```python
from build123d import *

# Parameters (mm, degrees)
BOX004_W          = 49.8
BOX004_H          = 30
BOX004_DEPTH      = 20
CYLINDER001_R     = 2
CYLINDER001_DEPTH = 54
CYLINDER_R        = 2
CYLINDER_DEPTH    = 54
BOX003_W          = 54
BOX003_H          = 30
BOX003_DEPTH      = 20
FILLET003_R       = 2
FILLET004_R       = 2
BOX002_W          = 30
BOX002_H          = 20
BOX002_DEPTH      = 2
FILLET002_R       = 3
BOX001_W          = 30
BOX001_H          = 40
BOX001_DEPTH      = 2
FILLET001_R       = 3
BOX_W             = 50
BOX_H             = 100
BOX_DEPTH         = 2
FILLET_R          = 3


with BuildPart() as cub004:
    # Box004 → Box004 (new body)
    with BuildSketch(Plane(origin=(2.1, 0, 0), x_dir=(1, 0, 0), z_dir=(0, 0, 1))):
        with Locations((24.9, 15)):
            Rectangle(BOX004_W, BOX004_H)
    extrude(amount=BOX004_DEPTH)


with BuildPart() as cilindre001:
    # Cylinder001 → Cylinder001 (new body)
    with BuildSketch(Plane(origin=(0, 23, 11), x_dir=(0, 0, -1), z_dir=(1, 0, 0))):
        Circle(CYLINDER001_R)
    extrude(amount=CYLINDER001_DEPTH)


with BuildPart() as cilindre:
    # Cylinder → Cylinder (new body)
    with BuildSketch(Plane(origin=(0, 7, 11), x_dir=(0, 0, -1), z_dir=(1, 0, 0))):
        Circle(CYLINDER_R)
    extrude(amount=CYLINDER_DEPTH)


with BuildPart() as fillet004:
    # Box003 → Box003 (new body)
    with BuildSketch(Plane.XY):
        with Locations((27, 15)):
            Rectangle(BOX003_W, BOX003_H)
    extrude(amount=BOX003_DEPTH)

    # Cut002: cut Cilindre
    add(cilindre.part, mode=Mode.SUBTRACT)

    # Cut003: cut Cilindre001
    add(cilindre001.part, mode=Mode.SUBTRACT)

    # Cut004: cut Cub004
    add(cub004.part, mode=Mode.SUBTRACT)

    # Fillet003
    fillet003_edges = [fillet004.edges().sort_by_distance(p)[0] for p in [
        (54, 15, 0),
    ]]
    fillet(fillet003_edges, radius=FILLET003_R)

    # Fillet004
    fillet004_edges = [fillet004.edges().sort_by_distance(p)[0] for p in [
        (0, 15, 0),
    ]]
    fillet(fillet004_edges, radius=FILLET004_R)


with BuildPart() as fillet004_1:
    # Fillet004 placement: moved
    add(fillet004.part.moved(Location((-2, 0, 0))))


with BuildPart() as fillet002:
    # Box002 → Box002 (new body)
    with BuildSketch(Plane(origin=(10, 70, 0), x_dir=(1, 0, 0), z_dir=(0, 0, 1))):
        with Locations((15, 10)):
            Rectangle(BOX002_W, BOX002_H)
    extrude(amount=BOX002_DEPTH)

    # Fillet002
    fillet002_edges = [fillet002.edges().sort_by_distance(p)[0] for p in [
        (10, 70, 1),
        (10, 90, 1),
        (40, 70, 1),
        (40, 90, 1),
    ]]
    fillet(fillet002_edges, radius=FILLET002_R)


with BuildPart() as fillet001:
    # Box001 → Box001 (new body)
    with BuildSketch(Plane(origin=(10, 10, 0), x_dir=(1, 0, 0), z_dir=(0, 0, 1))):
        with Locations((15, 20)):
            Rectangle(BOX001_W, BOX001_H)
    extrude(amount=BOX001_DEPTH)

    # Fillet001
    fillet001_edges = [fillet001.edges().sort_by_distance(p)[0] for p in [
        (10, 10, 1),
        (10, 50, 1),
        (40, 10, 1),
        (40, 50, 1),
    ]]
    fillet(fillet001_edges, radius=FILLET001_R)


with BuildPart() as fusion001:
    # Box → Box (new body)
    with BuildSketch(Plane.XY):
        with Locations((25, 50)):
            Rectangle(BOX_W, BOX_H)
    extrude(amount=BOX_DEPTH)

    # Fillet
    fillet_edges = [fusion001.edges().sort_by_distance(p)[0] for p in [
        (0, 100, 1),
        (50, 100, 1),
    ]]
    fillet(fillet_edges, radius=FILLET_R)

    # Cut: cut Fillet001
    add(fillet001.part, mode=Mode.SUBTRACT)

    # Cut001: cut Fillet002
    add(fillet002.part, mode=Mode.SUBTRACT)

    # Fusion: union Fillet004
    add(fillet004_1.part)


solid = fusion001.part
```
Build history of the part. All positions in model axes, mm. A direction names the side the tool comes from. Give positions to 0.01 mm unless a question says otherwise; leave off trailing zeros. Loops run counter-clockwise (first coordinate to the right, second up) from the corner with the lowest first, then second, coordinate; pieces in that order, holes last.
1) Band-saw the part on B-B on y = 23. List the corners of the cut face in (x, z), then the cut area to 3 significant figures.
Values follow:
outline: (-2, 2) arc R2 ccw to (0, 0) - (10, 0) - (10, 2) - (0.1, 2) - (0.1, 9) - (-2, 9) - close; (-2, 13) - (0.1, 13) - (0.1, 20) - (-2, 20) - close; (40, 0) - (50, 0) arc R2 ccw to (52, 2) - (52, 9) - (49.9, 9) - (49.9, 2) - (40, 2) - close; (49.9, 13) - (52, 13) - (52, 20) - (49.9, 20) - close
area: 105 mm2
2) Band-saw the part on C-C on x = 27. List the corners of the cut face in (y, z).
Values follow:
outline: (0, 0) - (10, 0) - (10, 2) - (0, 2) - close; (50, 0) - (70, 0) - (70, 2) - (50, 2) - close; (90, 0) - (100, 0) - (100, 2) - (90, 2) - close
3) Band-saw the part on D-D on z = 11. List the corners of the cut face in (x, y).
Values follow:
outline: (-2, 0) - (0.1, 0) - (0.1, 5) - (-2, 5) - close; (-2, 9) - (0.1, 9) - (0.1, 21) - (-2, 21) - close; (-2, 25) - (0.1, 25) - (0.1, 30) - (-2, 30) - close; (49.9, 0) - (52, 0) - (52, 5) - (49.9, 5) - close; (49.9, 9) - (52, 9) - (52, 21) - (49.9, 21) - close; (49.9, 25) - (52, 25) - (52, 30) - (49.9, 30) - close
4) Probe line 1 along Y through (x, z) = (50.5, 11); line 2 along Z through (x, y) = (0, 7); line 3 along X through (y, z) = (10.5, 17.25). List the from-to ranges inside material, lowest first.
Values follow:
line 1: y = 0 to 5, 9 to 21, 25 to 30
line 2: z = 0 to 9, 13 to 20
line 3: x = -2 to 0.1, 49.9 to 52
5) 3-axis set-ups, long thin cutter, end or side, ignore diameter. For faces 4 (the face through (24.9, 0, 1.8)), 5 (the face through (50, 63, 1)), 6 (the face through (-0.965, 8.352, 12.474)), 7 (the face through (39.1, 10.86, 1.01)), 8 (the face through (0.1, 15, 11)): which of +Z, -Z, +X, -X, +Y, -Y reach the whole face in a straight line?
Values follow:
face 4: +Z, -Z, +X, -X, -Y
face 5: +Z, -Z, +X, +Y
face 6: +X, -X
face 7: +Z, -Z
face 8: +Z, +Y, -Y
6) Two-plate mould, pull along Z, no slides. Class faces 1 (the face through (10, 30, 1)), 2 (the face through (-1.43, 15.21, 0.6)), 3 (the face through (-1, 21.8, 12.6)): released by +Z, released by -Z, zero draft, split by the parting line, or undercut.
Values follow:
face 1: zero draft
face 2: released by -Z
face 3: undercut
7) Drop flat-ended pins along their axis: P1, Ø2, axis at y = 78, z = 0.5, coming from the +X side; P2, Ø2, axis at y = 67.5, z = 1.5, coming from the -X side; P3, Ø0.6, axis at x = 50.5, z = 14, coming from the +Y side; P4, Ø15, axis at x = 31.5, y = 27.5, coming from the +Z side. Give the stop position or say it passes through.
Values follow:
P1: stops at x = 50
P2: stops at x = 0
P3: stops at y = 30
P4: passes through
8) Band-saw the part on A-A on z = 3. List the corners of the cut face in (x, y), then the cut area to 3 significant figures.
Values follow:
outline: (-2, 0) - (0.1, 0) - (0.1, 30) - (-2, 30) - close; (49.9, 0) - (52, 0) - (52, 30) - (49.9, 30) - close
area: 126 mm2
